```python
from build123d import *

# Parameters (mm, degrees)
SKETCH1_R      = 21
EXTRUDE1_DEPTH = 16
SKETCH5_R      = 1.75
EXTRUDE2_DEPTH = 1
SKETCH6_R      = 5
EXTRUDE3_DEPTH = 1
SKETCH7_R      = 3.75
EXTRUDE4_DEPTH = 11


with BuildPart() as part:
    # Sketch1 → Extrude1 (new body)
    with BuildSketch(Plane(origin=(0, 0, 0), x_dir=(1, 0, 0), z_dir=(0, 1, 0))):
        with Locations(Location((0, 0, 0), (0, 0, 270))):
            Circle(SKETCH1_R)
    extrude(amount=EXTRUDE1_DEPTH)

    # Sketch5 → Extrude2 (add)
    with BuildSketch(Plane(origin=(0, 16, 0), x_dir=(-1, 0, 0), z_dir=(0, 1, 0))):
        with BuildLine():
            Line((19.416487839, 8), (27.425754866, 2.468505292))
            ThreePointArc((27.425754866, 2.468505292), (28.720914222, 0), (27.425754866, -2.468505292))
            Line((27.425754866, -2.468505292), (19.416487839, -8))
            Line((19.416487839, -8), (-19.416487839, -8))
            Line((-19.416487839, -8), (-27.425754866, -2.468505292))
            ThreePointArc((-27.425754866, -2.468505292), (-28.720914222, 0), (-27.425754866, 2.468505292))
            Line((-27.425754866, 2.468505292), (-19.416487839, 8))
            Line((-19.416487839, 8), (19.416487839, 8))
        make_face()
        with Locations(Location((25.5, 0, 0), (0, 0, 90))):
            Circle(SKETCH5_R, mode=Mode.SUBTRACT)
        with Locations(Location((-25.5, 0, 0), (0, 0, 90))):
            Circle(SKETCH5_R, mode=Mode.SUBTRACT)
    extrude(amount=-EXTRUDE2_DEPTH)

    # Sketch6 → Extrude3 (add)
    with BuildSketch(Plane(origin=(0, 16, 0), x_dir=(-1, 0, 0), z_dir=(0, 1, 0))):
        with Locations(Location((0, 0, 0), (0, 0, 90))):
            Circle(SKETCH6_R)
    extrude(amount=EXTRUDE3_DEPTH)

    # Sketch7 → Extrude4 (add)
    with BuildSketch(Plane(origin=(0, 17, 0), x_dir=(-1, 0, 0), z_dir=(0, 1, 0))):
        with Locations(Location((0, 0, 0), (0, 0, 90))):
            Circle(SKETCH7_R)
    extrude(amount=EXTRUDE4_DEPTH)


solid = part.part
```
The model under review builds one solid part; all positions refer to its coordinate system, in mm. A direction names the side the tool comes from. Give positions to 0.01 mm unless a question says otherwise; leave off trailing zeros. Write each loop counter-clockwise with the first axis right and the second up, starting at its lowest first coordinate (ties: lowest second). Pieces come first, ordered by that corner, then holes. Notation, with made-up numbers: M 28.5,-39 L 54.5,-39 A8 cw 54.5,-31 Z; hole C -6.5,86 d2. An arc over 180 degrees is marked long. Write item = value, one per line. Start each with the question number.
Q1. Mouldability with a two-part tool opening along Z and no side actions: class faces 1 (the face through (23.37, 15.51, -5.27)), 2 (the face through (0, 28, 0)), 3 (the face through (27.235, 15.507, -0.228)) as released by +Z, released by -Z, zero draft, split by the parting line, or undercut.
Q2. For line 1 (X direction, y = 15.5, z = 0); line 2 (Y direction, x = 23, z = -5); line 3 (Y direction, x = 13, z = 3.5), list the stretches that pass through material, from the lowest coordinate up.
Q3. We need section C-C (x = 25.5). State the section outline as (y, z) points, plus the area to 3 significant figures.
Q4. We need section D-D (y = 2.25). State the section outline as (x, z) points, plus the area to 3 significant figures.
Q5. Machinability: for faces 4 (the face through (-4.88, 16.49, -1.08)), 5 (the face through (6.31, 7.89, 20.03)), 6 (the face through (-23.765, 15.507, -0.228)), which of the approach directions +Z, -Z, +X, -X, +Y, -Y give a long, thin tool a straight path to every point of the face, cutting with its end or side? Answer none if there is none.
Q6. We need section A-A (z = 0). State the section outline as (x, y) points, plus the area to 3 significant figures.
Q7. We need section B-B (x = 0). State the section outline as (y, z) points, plus the area to 4 significant figures.
Q8. Clearance check with flat-ended pins moving along their axes: pin 1 (4 mm diameter, centred on x = -2, z = -6.5, fed in from +Y); pin 2 (8 mm diameter, centred on x = 13, y = 14, fed in from -Z); pin 3 (1 mm diameter, centred on x = 11, z = -15.5, fed in from +Y). State where each tip first meets the part, or that it passes through.
Result set:
q1.face_1 = released by -Z
q1.face_2 = zero draft
q1.face_3 = undercut
q2.line_1 = -28.72 to -27.25, -23.75 to 23.75, 27.25 to 28.72
q2.line_2 = 15 to 16
q2.line_3 = 0 to 16
q3.outline = M 15,-3.8 L 16,-3.8 L 16,-1.75 L 15,-1.75 Z; M 15,1.75 L 16,1.75 L 16,3.8 L 15,3.8 Z
q3.area = 4.10 mm2
q4.outline = C 0,0 d42
q4.area = 1,390 mm2
q5.face_4 = +Y
q5.face_5 = -Y
q5.face_6 = +Y, -Y
q6.outline = M -28.72,15 L -27.25,15 L -27.25,16 L -28.72,16 Z; M -23.75,15 L -21,15 L -21,0 L 21,0 L 21,15 L 23.75,15 L 23.75,16 L 5,16 L 5,17 L 3.75,17 L 3.75,28 L -3.75,28 L -3.75,17 L -5,17 L -5,16 L -23.75,16 Z; M 27.25,15 L 28.72,15 L 28.72,16 L 27.25,16 Z
q6.area = 773 mm2
q7.outline = M 0,-21 L 16,-21 L 16,-5 L 17,-5 L 17,-3.75 L 28,-3.75 L 28,3.75 L 17,3.75 L 17,5 L 16,5 L 16,21 L 0,21 Z
q7.area = 764.5 mm2
q8.pin_1 = 17
q8.pin_2 = -18.97
q8.pin_3 = 16
